from build123d import *

# Parameters (mm, degrees)
F0_W     = 20
F0_H     = 20
F1_DEPTH = 310
F2_W     = 20
F2_H     = 20
F3_DEPTH = 260
F4_W     = 20
F4_H     = 20
F5_DEPTH = 215
F6_W     = 20
F6_H     = 20
F7_DEPTH = 580
F8_R     = 5
F9_DEPTH = 620


with BuildPart() as f1:
    # F0 (on Front) → F1 (new body, symmetric)
    with BuildSketch(Plane.XZ):
        with Locations((10, 260)):
            Rectangle(F0_W, F0_H)
    extrude(amount=F1_DEPTH, both=True)

    # F2 (on face) → F3 (join)
    with BuildSketch(Plane(origin=(0, 0, 250), x_dir=(1, 0, 0), z_dir=(0, 0, -1))):
        with Locations((10, 300)):
            Rectangle(F2_W, F2_H)
        with Locations((10, -300)):
            Rectangle(F2_W, F2_H)
    extrude(amount=F3_DEPTH)



with BuildPart() as f1b:
    # F0 (on Front) → F1, piece 2 (new body, symmetric)
    with BuildSketch(Plane.XZ):
        with Locations((245, 260)):
            Rectangle(F0_W, F0_H)
    extrude(amount=F1_DEPTH, both=True)

    # F2 (on face) → F3, piece 2 (join)
    with BuildSketch(Plane(origin=(0, 0, 250), x_dir=(1, 0, 0), z_dir=(0, 0, -1))):
        with Locations((245, -300)):
            Rectangle(F2_W, F2_H)
        with Locations((245, 300)):
            Rectangle(F2_W, F2_H)
    extrude(amount=F3_DEPTH)


with BuildPart() as f1_1:
    add(f1.part)

    add(f1b.part)  # F5 merges F1b
    # F4 (on face) → F5 (join, through all)
    with BuildSketch(Plane(origin=(235, 0, 0), x_dir=(0, -1, 0), z_dir=(-1, 0, 0))):
        with Locations((-300, 260)):
            Rectangle(F4_W, F4_H)
        with Locations((-300, 0)):
            Rectangle(F4_W, F4_H)
        with Locations((300, 0)):
            Rectangle(F4_W, F4_H)
        with Locations((300, 260)):
            Rectangle(F4_W, F4_H)
    extrude(amount=F5_DEPTH)

    # F6 (on face) → F7 (join, through all)
    with BuildSketch(Plane(origin=(0, -290, 0), x_dir=(-1, 0, 0), z_dir=(0, 1, 0))):
        with Locations((-10, 55)):
            Rectangle(F6_W, F6_H)
    extrude(amount=F7_DEPTH)

    # F8 (on face) → F9 (cut, through all)
    with BuildSketch(Plane(origin=(0, 310, 0), x_dir=(-1, 0, 0), z_dir=(0, 1, 0))):
        with Locations((-40, 0)):
            Circle(F8_R)
    extrude(amount=-F9_DEPTH, mode=Mode.SUBTRACT)


solid = f1_1.part
Input: part model. Units: mm. Frame: model coordinates. A direction names the side the tool comes from. Give positions to 0.01 mm unless a question says otherwise; leave off trailing zeros. Loops run counter-clockwise (first coordinate to the right, second up) from the corner with the lowest first, then second, coordinate; pieces in that order, holes last. Notation, with made-up numbers: M 44.25,45 L 67.25,45 A12 ccw 67.25,59 Z; hole C 81,-5 d8. An arc over 180 degrees is marked long. Use one line per item in the form item = value.
1. Section query C-C, the plane y = 1. Return the cut outline in (x, z), and give its area (3 significant figures).
Numbers:
outline = M 0,45 L 20,45 L 20,65 L 0,65 Z; M 0,250 L 20,250 L 20,270 L 0,270 Z; M 235,250 L 255,250 L 255,270 L 235,270 Z
area = 1,200 mm²
2. Line query: L1, parallel to Z at x = 40, y = 297; L2, parallel to Y at x = 188.5, z = 250.5; L3, parallel to Z at x = 14.5, y = 96.5. Output: solid intervals per line, ascending.
Numbers:
L1 = -10 to -5, 5 to 10, 250 to 270
L2 = -310 to -290, 290 to 310
L3 = 45 to 65, 250 to 270
3. Reachability of faces 4 (the face through (10, -4, 65)), 5 (the face through (129, 300, 250)), 6 (the face through (245, -4, 250)), 7 (the face through (129, -290, 260)) from +Z, -Z, +X, -X, +Y, -Y: full face, straight path, thin tool, end or side. Return the list, or none.
Numbers:
face_4 = +X, -X
face_5 = +Y, -Y
face_6 = -Z, +X, -X
face_7 = +Z, -Z
4. Section query B-B, the plane z = 53. Return the cut outline in (x, y).
Numbers:
outline = M 0,-310 L 20,-310 L 20,310 L 0,310 Z; M 235,-310 L 255,-310 L 255,-290 L 235,-290 Z; M 235,290 L 255,290 L 255,310 L 235,310 Z
5. Section query A-A, the plane x = 148. Return the cut outline in (y, z).
Numbers:
outline = M -310,-10 L -290,-10 L -290,10 L -310,10 Z; M -310,250 L -290,250 L -290,270 L -310,270 Z; M 290,-10 L 310,-10 L 310,10 L 290,10 Z; M 290,250 L 310,250 L 310,270 L 290,270 Z
6. First-contact query: pin 1 (10 mm diameter, centred on y = 141.5, z = 256, fed in from -X); pin 2 (12 mm diameter, centred on y = -189.5, z = 57.5, fed in from +X); pin 3 (16 mm diameter, centred on x = 5.5, y = 64.5, fed in from -Z). Flat tips, straight axial feed; report the tip coordinate or a pass-through.
Numbers:
pin_1 = 0
pin_2 = 20
pin_3 = 45
7. Pull-direction query (Z, two-part tool) for faces 1 (the face through (15, 24, 270)), 2 (the face through (20, 4, 260)), 3 (the face through (235, 300, 132)); classes: released by +Z, released by -Z, zero draft, split by the parting line, or undercut.
Numbers:
face_1 = released by +Z
face_2 = zero draft
face_3 = undercut
